The model under review builds one solid part; all positions refer to its coordinate system, in mm. Face numbers are marked on the shaded views. A direction names the side the tool comes from. Round coordinates to 2 decimals unless told otherwise and drop trailing zeros. Order: outer loops, then holes, each group sorted by start corner. A loop starts at its lowest first (then second) coordinate and runs counter-clockwise, first axis right, second up. Notation, with made-up numbers: M 35.5,-29 L 42.5,-29 A24 cw 42.5,10 Z; hole C 54,61.25 d5. An arc over 180 degrees is marked long. One line per item, written item: value. Start each with the question number.
from build123d import *

# Parameters (mm, degrees)
EXTRUSION1_DEPTH        = 17.5
CONG_1_R                = 6
ESQUISSE2_R             = 3
ENL_V_MAT_EXTRU_1_DEPTH = 20
ENL_V_MAT_EXTRU_6_DEPTH = 35
ESQUISSE4_W             = 10
ESQUISSE4_H             = 4
ENL_V_MAT_EXTRU_7_DEPTH = 12.0000001


with BuildPart() as part:
    # Esquisse1 → Extrusion1 (new body, symmetric)
    with BuildSketch(Plane.XY):
        with BuildLine():
            Line((8, 2), (8, 0))
            ThreePointArc((8, 0), (0, -8), (-8, 0))
            Line((-8, 0), (-8, 3))
            Line((-8, 3), (-11, 3))
            Line((-11, 3), (-11, 0))
            ThreePointArc((-11, 0), (0, -11), (11, 0))
            Line((11, 0), (11, 2))
            ThreePointArc((11, 2), (11.878679656, 4.121320344), (14, 5))
            Line((14, 5), (28, 5))
            Line((28, 5), (28, 8))
            Line((28, 8), (14, 8))
            ThreePointArc((14, 8), (9.757359313, 6.242640687), (8, 2))
        make_face()
    extrude(amount=EXTRUSION1_DEPTH, both=True)

    # Congé1
    cong_1_edges = [part.edges().sort_by_distance(p)[0] for p in [
        (28, 6.5, -17.5),
        (28, 6.5, 17.5),
    ]]
    fillet(cong_1_edges, radius=CONG_1_R)

    # Esquisse2 → Enlèv. mat.-Extru.1 (cut, through all)
    with BuildSketch(Plane(origin=(0, 8, 0), x_dir=(-1, 0, 0), z_dir=(0, 1, 0))):
        with Locations(Location((-19, 0, 0), (0, 0, 90))):  # turned: the seam where the file's is
            Circle(ESQUISSE2_R)
    extrude(amount=-ENL_V_MAT_EXTRU_1_DEPTH, mode=Mode.SUBTRACT)

    # Esquisse3 → Enlèv. mat.-Extru.6 (cut)
    with BuildSketch(Plane.ZY.offset(8)):
        with BuildLine():
            Line((-9, 8), (-17.5, 8))
            Line((-17.5, 8), (-17.5, -0.5))
            ThreePointArc((-17.5, -0.5), (-15.01040764, 5.51040764), (-9, 8))
        make_face()
        with BuildLine():
            Line((17.5, 8), (17.5, -0.5))
            ThreePointArc((17.5, -0.5), (15.01040764, 5.51040764), (9, 8))
            Line((9, 8), (17.5, 8))
        make_face()
    extrude(amount=ENL_V_MAT_EXTRU_6_DEPTH, mode=Mode.SUBTRACT)

    # Esquisse4 → Enlèv. mat.-Extru.7 (cut, through all)
    with BuildSketch(Plane(origin=(0, 0, 0), x_dir=(0, 0, -1), z_dir=(1, 0, 0))):
        with Locations((0, 1)):
            Rectangle(ESQUISSE4_W, ESQUISSE4_H)
    extrude(amount=-ENL_V_MAT_EXTRU_7_DEPTH, mode=Mode.SUBTRACT)


solid = part.part
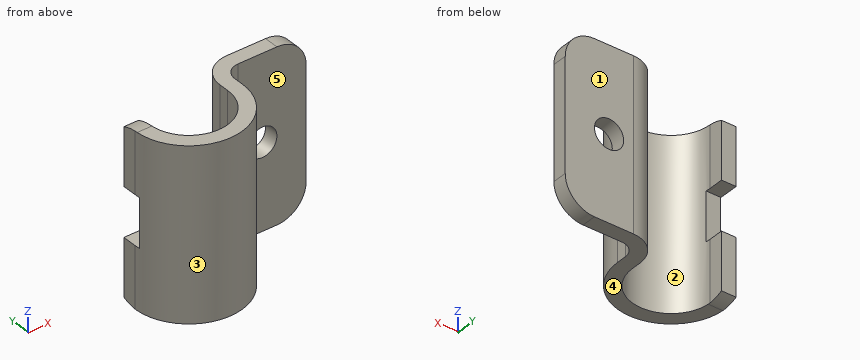
Item 1: Consider section D-D, the plane x = 14.5. Give the boundary of the cut face in (y, z), then the cut area to 3 significant figures.
Item 2: Machinability: for the marked faces 4 and 5, which of the approach directions +Z, -Z, +X, -X, +Y, -Y give a long, thin tool a straight path to every point of the face, cutting with its end or side? Answer none if there is none.
Item 3: Consider section A-A, the plane x = 19. Give the boundary of the cut face in (y, z).
Item 4: Consider section C-C, the plane y = -5. Give the boundary of the cut face in (x, z) (3 decimals).
Item 5: Clearance check with flat-ended pins moving along their axes: P1, Ø10, axis at y = 3, z = 1, coming from the +X side; P2, Ø1, axis at y = -2.5, z = 7.5, coming from the -X side; P3, Ø2, axis at y = -3.5, z = 0, coming from the +X side; P4, Ø2.5, axis at x = -8.5, y = 2, coming from the -Z side. State where each tip first meets the part, or that it passes through.
Item 6: The part is to be moulded in two halves that separate along X. For the marked faces 1, 2 and 3, say which applies: pulls with the +X half, pulls with the -X half, needs draft (parallel to the pull), parting line crosses it, or undercut.
Item 7: Consider section B-B, the plane z = 0. Give the boundary of the cut face in (x, y).
Item 8: Wall thickness on L1, parallel to Y at x = 14, z = 1; L2, parallel to X at y = 7.4, z = 0; L3, parallel to X at y = 6.8, z = 0: over which ranges is each line inside the solid? List them lowest first.
Computed:
1. outline: M 5,-17.5 L 8,-17.5 L 8,17.5 L 5,17.5 Z
1. area: 105 mm^2
2. face 4: -Z, +X, -X, +Y, -Y
2. face 5: +Z, -Z, +X, -Y
3. outline: M 5,-17.5 L 8,-17.5 L 8,-3 L 5,-3 Z; M 5,3 L 8,3 L 8,17.5 L 5,17.5 Z
4. outline: M -9.798,-17.5 L -6.245,-17.5 L -6.245,17.5 L -9.798,17.5 Z; M 6.245,-17.5 L 9.798,-17.5 L 9.798,17.5 L 6.245,17.5 Z
5. P1: stops at x = 28
5. P2: stops at x = -10.82
5. P3: stops at x = 10.71
5. P4: stops at z = -17.41
6. face 1: needs draft
6. face 2: undercut
6. face 3: parting line crosses it
7. outline: M -10.95,-1 A11 ccw 11,0 L 11,2 A3 cw 14,5 L 16,5 L 16,8 L 14,8 A6 ccw 8,2 L 8,0 A8 cw -7.94,-1 Z; M 22,5 L 28,5 L 28,8 L 22,8 Z
8. L1: y = 5 to 8
8. L2: x = 11.38 to 16, 22 to 28
8. L3: x = 10.4 to 16, 22 to 28
